from build123d import *

# Parameters (mm, degrees)
F0_W     = 114.3
F0_H     = 63.5
F1_DEPTH = 12.7
F4_DEPTH = 12.7
F5_DEPTH = 25.4
F6_DEPTH = 38.1


with BuildPart() as f1:
    # F0 (on Top) → F1 (new body)
    with BuildSketch(Plane.XY):
        with Locations((57.15, 31.75)):
            Rectangle(F0_W, F0_H)
    extrude(amount=F1_DEPTH)

    # F3 (on offset) → F4 (join)
    with BuildSketch(Plane.XY.offset(12.7)):
        Polygon((12.7, 19.05), (31.75, 19.05), (38.1, 19.05), (38.1, 6.35), (76.2, 6.35), (76.2, 19.05), (82.55, 19.05), (101.6, 19.05), (101.6, 50.8), (12.7, 50.8), align=None)
    extrude(amount=F4_DEPTH)

    # F3 (on offset) → F5 (join)
    with BuildSketch(Plane.XY.offset(12.7)):
        Polygon((0, 50.8), (0, 0), (31.75, 0), (31.75, 19.05), (12.7, 19.05), (12.7, 50.8), align=None)
        Polygon((82.55, 19.05), (82.55, 0), (114.3, 0), (114.3, 50.8), (101.6, 50.8), (101.6, 19.05), align=None)
    extrude(amount=F5_DEPTH)

    # F3 (on offset) → F6 (join)
    with BuildSketch(Plane.XY.offset(12.7)):
        Polygon((31.75, 19.05), (31.75, 0), (82.55, 0), (82.55, 19.05), (76.2, 19.05), (76.2, 6.35), (38.1, 6.35), (38.1, 19.05), align=None)
    extrude(amount=F6_DEPTH)


solid = f1.part
Could you check a few things on this model? Use its own coordinates, in mm. A direction names the side the tool comes from. Round coordinates to 2 decimals unless told otherwise and drop trailing zeros. Write each loop counter-clockwise with the first axis right and the second up, starting at its lowest first coordinate (ties: lowest second). Pieces come first, ordered by that corner, then holes. Notation, with made-up numbers: (-8.75, -31) -> (20.25, -31) arc R25 ccw to (20.25, -12) -> close; hole circle Ø8 at (-24, 58.25). An arc over 180 degrees is marked (long way). Use a Markdown table: item, result.
1. If we section it at A-A (x = 30.5): List the corners of the cut face in (y, z) for me, then the cut area to 3 significant figures.
Answer key:
| item | result |
|---|---|
| outline | (0, 0) -> (63.5, 0) -> (63.5, 12.7) -> (50.8, 12.7) -> (50.8, 25.4) -> (19.05, 25.4) -> (19.05, 38.1) -> (0, 38.1) -> close |
| area | 1,690 mm^2 |
2. Which directions (+Z, -Z, +X, -X, +Y, -Y) give clear straight access to the entire face, cutting with the end or side of a thin tool? Please do faces 1 (the face through (12, 20, 38.1)), 2 (the face through (82.55, 9, 44)), 3 (the face through (114.3, 24, 19)), 4 (the face through (38.1, 13, 38)), 5 (the face through (58, 50.8, 22)).
Answer key:
| item | result |
|---|---|
| face 1 | +Z, -X, +Y, -Y |
| face 2 | +Z, +X, +Y, -Y |
| face 3 | +Z, -Z, +X, +Y, -Y |
| face 4 | +Z, +Y |
| face 5 | +Z, +X, -X, +Y |
3. If we section it at B-B (y = 12): List the corners of the cut face in (x, z) for me.
Answer key:
| item | result |
|---|---|
| outline | (0, 0) -> (114.3, 0) -> (114.3, 38.1) -> (82.55, 38.1) -> (82.55, 50.8) -> (76.2, 50.8) -> (76.2, 25.4) -> (38.1, 25.4) -> (38.1, 50.8) -> (31.75, 50.8) -> (31.75, 38.1) -> (0, 38.1) -> close |
4. If we section it at D-D (z = 22): List the corners of the cut face in (x, y) for me.
Answer key:
| item | result |
|---|---|
| outline | (0, 0) -> (114.3, 0) -> (114.3, 50.8) -> (0, 50.8) -> close |
5. We'd pull the mould along X, two halves only. Please class faces 6 (the face through (28, 19.05, 35)), 7 (the face through (56, 63.5, 6)), 8 (the face through (0, 25, 19)): +X half, -X half, draft (parallel to the pull), parting line (faces both ways), or undercut.
Answer key:
| item | result |
|---|---|
| face 6 | undercut |
| face 7 | draft |
| face 8 | -X half |
6. If we section it at C-C (z = 41.5): List the corners of the cut face in (x, y) for me, then the cut area to 3 significant figures.
Answer key:
| item | result |
|---|---|
| outline | (31.75, 0) -> (82.55, 0) -> (82.55, 19.05) -> (76.2, 19.05) -> (76.2, 6.35) -> (38.1, 6.35) -> (38.1, 19.05) -> (31.75, 19.05) -> close |
| area | 484 mm^2 |
7. Please list where these lines run through material, in increasing order: probe 1 along X at (y, z) = (7.5, 31); probe 2 along Z at (x, y) = (84, 42.5); probe 3 along Y at (x, z) = (39.5, 22).
Answer key:
| item | result |
|---|---|
| probe 1 | x = 0 to 38.1, 76.2 to 114.3 |
| probe 2 | z = 0 to 25.4 |
| probe 3 | y = 0 to 50.8 |
8. For pin 1 Ø4 at (x, y) = (80, 49) entering from +Z; pin 2 Ø9.5 at (x, y) = (13.5, 20) entering from +Z; pin 3 Ø6.5 at (x, y) = (85, 54.5) entering from +Z; pin 4 Ø4 at (y, z) = (30.5, 30.5) entering from -X, each with a flat end and sliding along its axis, tell me the tip position at first contact or that it passes through.
Answer key:
| item | result |
|---|---|
| pin 1 | stops at z = 25.4 |
| pin 2 | stops at z = 38.1 |
| pin 3 | stops at z = 12.7 |
| pin 4 | stops at x = 0 |
